from build123d import *

# Parameters (mm, degrees)
SKETCH_2_W          = 25
SKETCH_2_H          = 15
SKETCH_2_R          = 1.6
EXTRUDE_1_DEPTH     = 2
SKETCH_3_W          = 1.5
SKETCH_3_H          = 10
SKETCH_3_W_2        = 2
EXTRUDE_2_DEPTH     = 7
FILLET_1_R          = 2
SKETCH_4_R          = 1.65
CUT_EXTRUDE_1_DEPTH = 28.608875385


with BuildPart() as part:
    # 草图2 → 凸台-拉伸1 (new body)
    with BuildSketch(Plane.XY):
        Rectangle(SKETCH_2_W, SKETCH_2_H)
        with Locations((-8, -3.5)):
            Circle(SKETCH_2_R, mode=Mode.SUBTRACT)
        with Locations((8, -3.5)):
            Circle(SKETCH_2_R, mode=Mode.SUBTRACT)
    extrude(amount=EXTRUDE_1_DEPTH)

    # 草图3 → 凸台-拉伸2 (add)
    with BuildSketch(Plane.XY.offset(2)):
        with Locations((-11.75, 2.5)):
            Rectangle(SKETCH_3_W, SKETCH_3_H)
        with Locations((-2.5, 2.5)):
            Rectangle(SKETCH_3_W_2, SKETCH_3_H)
        with Locations((2.5, 2.5)):
            Rectangle(SKETCH_3_W_2, SKETCH_3_H)
        with Locations((11.75, 2.5)):
            Rectangle(SKETCH_3_W, SKETCH_3_H)
    extrude(amount=EXTRUDE_2_DEPTH)

    # 圆角1
    fillet_1_edges = [part.edges().sort_by_distance(p)[0] for p in [
        (-11.75, -2.5, 2),
        (-11.75, -2.5, 9),
        (-11.75, 7.5, 9),
        (-2.5, -2.5, 2),
        (-2.5, -2.5, 9),
        (-2.5, 7.5, 9),
        (2.5, -2.5, 2),
        (2.5, -2.5, 9),
        (2.5, 7.5, 9),
        (11.75, -2.5, 2),
        (11.75, 7.5, 9),
        (11.75, -2.5, 9),
        (12.5, -7.5, 1),
        (-12.5, -7.5, 1),
    ]]
    fillet(fillet_1_edges, radius=FILLET_1_R)

    # 草图4 → 切除-拉伸1 (cut, through all)
    with BuildSketch(Plane.ZY.offset(12.5)):
        with Locations(Location((6.2, 4, 0), (0, 0, 270))):
            Circle(SKETCH_4_R)
    extrude(amount=-CUT_EXTRUDE_1_DEPTH, mode=Mode.SUBTRACT)


solid = part.part
Here's how the part is built. I have some questions about the finished solid (model axes, mm). A direction names the side the tool comes from. Coordinates: 2 decimals unless noted, no trailing zeros. Order: outer loops, then holes, each group sorted by start corner. A loop starts at its lowest first (then second) coordinate and runs counter-clockwise, first axis right, second up.
Item 1: If we section it at A-A on z = 6.2: State how many separate pieces and enclosed holes the cut face has, plus the area to 3 significant figures.
Result sheet:
separate pieces: 8
enclosed holes: 0
area: 46.9 mm2
Item 2: For P1, Ø1.6, axis at x = 2.5, z = 6, coming from the -Y side; P2, Ø5, axis at x = -8, y = -3.5, coming from the +Z side; P3, Ø3, axis at y = 4, z = 6.2, coming from the +X side, each with a flat end and sliding along its axis, tell me the tip position at first contact or that it passes through.
Result sheet:
P1: stops at y = -2.5
P2: stops at z = 2
P3: passes through
Item 3: If we section it at B-B on x = 8: List the corners of the cut face in (y, z) for me.
Result sheet:
outline: (-7.5, 0) - (-5.1, 0) - (-5.1, 2) - (-7.5, 2) - close; (-1.9, 0) - (7.5, 0) - (7.5, 2) - (-1.9, 2) - close
Item 4: I need wall thicknesses on line 1 (X direction, y = 6.25, z = 3.75); line 2 (Z direction, x = 2.75, y = 4); line 3 (Z direction, x = 8.5, y = 1.5). Which ranges of each line are inside material? Lowest first, please.
Result sheet:
line 1: x = -12.5 to -11, -3.5 to -1.5, 1.5 to 3.5, 11 to 12.5
line 2: z = 0 to 4.55, 7.85 to 9
line 3: z = 0 to 2
Item 5: If we section it at D-D on z = 1.5: List the corners of the cut face in (x, y) for me, plus the area to 3 significant figures.
Result sheet:
outline: (-12.5, -5.5) arc R2 ccw to (-10.5, -7.5) - (10.5, -7.5) arc R2 ccw to (12.5, -5.5) - (12.5, 7.5) - (-12.5, 7.5) - close; hole circle Ø3.2 at (-8, -3.5); hole circle Ø3.2 at (8, -3.5)
area: 357 mm2
Item 6: For faces 4 (the face through (-12, -2.5, 5)), 5 (the face through (-1.5, 2.7, 4.7)), 6 (the face through (12.5, 2, 4)), which set-ups out of +Z, -Z, +X, -X, +Y, -Y let a thin tool reach every point of the face, with its end or its side?
Result sheet:
face 4: +Z, +X, -X, -Y
face 5: +Z, +Y, -Y
face 6: +Z, -Z, +X, +Y, -Y
Item 7: If we mould it in two halves opening along X, with no side actions, what happens to faces 1 (the face through (-12.5, 2, 4)), 2 (the face through (-11.76, 4.215, 7.836)), 3 (the face through (1.5, 2.7, 4.7))? For each: +X half, -X half, draft (parallel to the pull), parting line (faces both ways), or undercut.
Result sheet:
face 1: -X half
face 2: draft
face 3: undercut
Item 8: If we section it at C-C on y = -3.5: List the corners of the cut face in (x, z) for me.
Result sheet:
outline: (-12.5, 0) - (-9.6, 0) - (-9.6, 2) - (-11, 2) - (-11, 2.27) - (-12.5, 2.27) - close; (-6.4, 0) - (6.4, 0) - (6.4, 2) - (3.5, 2) - (3.5, 2.27) - (1.5, 2.27) - (1.5, 2) - (-1.5, 2) - (-1.5, 2.27) - (-3.5, 2.27) - (-3.5, 2) - (-6.4, 2) - close; (9.6, 0) - (12.5, 0) - (12.5, 2.27) - (11, 2.27) - (11, 2) - (9.6, 2) - close
